Study the drawing (mm; zero at the part's minimum x, y, z) and answer. A direction names the side the tool comes from. Give positions to 0.01 mm unless a question says otherwise; leave off trailing zeros. Order: outer loops, then holes, each group sorted by start corner. A loop starts at its lowest first (then second) coordinate and runs counter-clockwise, first axis right, second up.
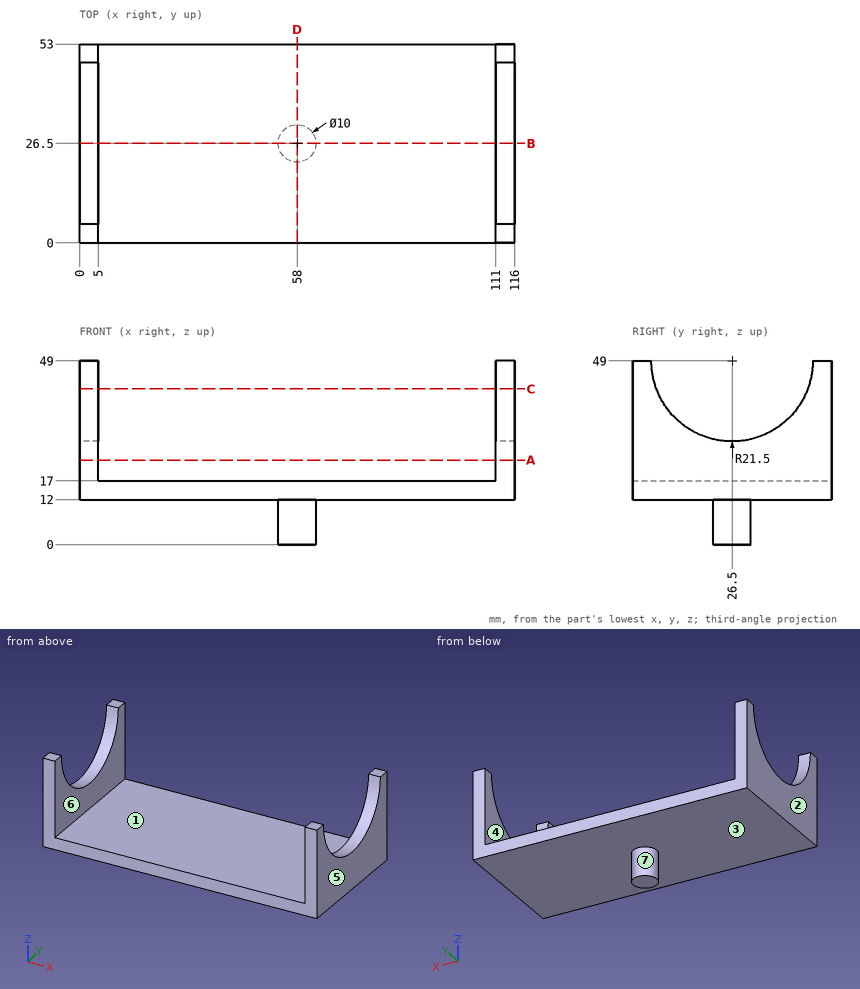
1) For a pull along X with two mould halves and no side action, classify the marked faces 1, 2, 3 and 4 as +X half, -X half, draft (parallel to the pull), parting line (faces both ways), or undercut.
Geometry says:
face 1: undercut
face 2: -X half
face 3: draft
face 4: undercut
2) Given P1, Ø16, axis at x = 75, y = 22, coming from the +Z side; P2, Ø8, axis at x = 81.5, y = 30, coming from the -Z side; P3, Ø5, axis at y = 22, z = 6, coming from the +X side, each flat-ended and moving along its own axis, determine where each tip first touches the part or whether it passes through.
Geometry says:
P1: stops at z = 17
P2: stops at z = 12
P3: stops at x = 62.58
3) A tool of negligible diameter and unlimited length cuts with its end or side. For the marked faces 5, 6 and 7, from which of +Z, -Z, +X, -X, +Y, -Y can it reach the whole face along a straight path? Write none if from no direction.
Geometry says:
face 5: +Z, -Z, +X, +Y, -Y
face 6: +Z, +Y, -Y
face 7: -Z
4) Find section B-B (y = 26.5). Write down the section's boundary in (x, z).
Geometry says:
outline: (0, 12) - (53, 12) - (53, 0) - (63, 0) - (63, 12) - (116, 12) - (116, 27.5) - (111, 27.5) - (111, 17) - (5, 17) - (5, 27.5) - (0, 27.5) - close
5) Find section D-D (x = 58). Write down the section's boundary in (y, z), then the cut area to 3 significant figures.
Geometry says:
outline: (0, 12) - (21.5, 12) - (21.5, 0) - (31.5, 0) - (31.5, 12) - (53, 12) - (53, 17) - (0, 17) - close
area: 385 mm2
6) Find section A-A (z = 22.5). Write down the section's boundary in (x, y).
Geometry says:
outline: (0, 0) - (5, 0) - (5, 53) - (0, 53) - close; (111, 0) - (116, 0) - (116, 53) - (111, 53) - close
7) Find section C-C (z = 41.5). Write down the section's boundary in (x, y), then the cut area to 3 significant figures.
Geometry says:
outline: (0, 0) - (5, 0) - (5, 6.35) - (0, 6.35) - close; (0, 46.65) - (5, 46.65) - (5, 53) - (0, 53) - close; (111, 0) - (116, 0) - (116, 6.35) - (111, 6.35) - close; (111, 46.65) - (116, 46.65) - (116, 53) - (111, 53) - close
area: 127 mm2
8) Straight lines are drawn through the part: probe 1 along X at (y, z) = (11, 25.5); probe 2 along Z at (x, y) = (32.5, 20.5); probe 3 along Z at (x, y) = (57, 28). For each, find the intervals that lie inside material, in ascending order.
Geometry says:
probe 1: x = 0 to 5, 111 to 116
probe 2: z = 12 to 17
probe 3: z = 0 to 17
